Autodesk Fusion 360 part; units mm, degrees
sketch "Esboço1" plane through (0, 0, 0) normal (0, 0, 1) x (1, 0, 0)
  line L0 (0, -15) -> (47.41, -15)
  arc A0 (47.41, -15) -> (47.41, 15) centre (47.41, 0) ccw
  line L1 (47.41, 15) -> (0, 15)
  arc A1 (0, 15) -> (0, -15) centre (0, 0) ccw
  line L2 (0, 0) -> (47.41, 0) construction
  line L3 (-15, 0) -> (62.41, 0) construction
  circle A2 centre (0, 0) radius 3.75
  circle A3 centre (18.25, 0) radius 1.875
  dimension "d1" = 15
  dimension "d4" = 77.41
  dimension "d5" = 7.5
  dimension "d6" = 18.25
  dimension "d7" = 3.75
extrude "Extrusão1" add sketch "Esboço1" along normal blind 5
sketch "Esboço2" plane through (0, 0, 5) normal (0, 0, 1) x (-1, 0, 0)
  circle A0 centre (-18.25, 0) radius 1.875
  circle A1 centre (0, 0) radius 3.75
  arc A2 (0, -15) -> (0, 15) centre (0, 0) ccw
  line L0 (0, 15) -> (-47.41, 15)
  arc A3 (-47.41, 15) -> (-47.41, -15) centre (-47.41, 0) ccw
  line L1 (-47.41, -15) -> (0, -15)
  line L2 (0, 10) -> (-36.5, 10)
  arc A4 (-36.5, 10) -> (-36.5, -10) centre (-36.5, 0) ccw
  line L3 (-36.5, -10) -> (0, -10)
  arc A5 (0, -10) -> (0, 10) centre (0, 0) ccw
  line L4 (0, 0) -> (-36.5, 0) construction
  dimension "d10" = 36.5
  dimension "d11" = 10
extrude "Extrusão2" cut sketch "Esboço2" against normal blind 3.5 contours L2 A4 L3 A5
hole "Furo1" at (36.5, 0, 1.5) direction (0, 0, -1) diameter 10 depth 0.75 tip angle 180
chamfer "Chanfro1" distance 0.75 angle 45 1 edges at (31.8384, 1.8081, 1.5)
chamfer "Chanfro2" distance 5 angle 45 4 edges at (23.705, 15, 0) (-15, 0, 0) (23.705, -15, 0) (62.41, 0, 0)
Build history of the part. All positions in model axes, mm. A direction names the side the tool comes from. Coordinates: 2 decimals unless noted, no trailing zeros. Order: outer loops, then holes, each group sorted by start corner. A loop starts at its lowest first (then second) coordinate and runs counter-clockwise, first axis right, second up. Notation, with made-up numbers: M 12,12 L 27,12 A17 cw 27,37 Z; hole C 5.5,49 d4. An arc over 180 degrees is marked long. One line per question, with ' | ' between items. Start each with the question number.
1. Mould opens along X. For faces 3 (the face through (57.72, -0.23, 0.31)), 4 (the face through (-3.746, -0.165, 0.74)), 5 (the face through (23.2, 10.2, 5)) say: +X half, -X half, draft (parallel to the pull), parting line (faces both ways), or undercut.
2. Wall check: line 1 along X through (y, z) = (-1, 1.2); line 2 along Y through (x, z) = (18.25, 0.65) (3 decimals); line 3 along Z through (x, y) = (9.5, 9.5). Give the ranges that are in metal, low to high. Write a range as [from, to].
3. Tool access for faces 1 (the face through (19, -2, 1.5)), 2 (the face through (23, -13, 3)): list every direction of +Z, -Z, +X, -X, +Y, -Y with a clear straight run to the whole face (end or side of a thin tool).
4. Flat gauge pins, fed straight in: P1, Ø8, axis at x = 36.5, y = 0, coming from the -Z side; P2, Ø1.5, axis at y = 8, z = 1.5, coming from the +X side; P3, Ø3.5, axis at x = 18.25, y = 0, coming from the +Z side; P4, Ø1, axis at x = 8, z = 1.5, coming from the -Y side. Where does each tip first touch, or does it go through?
5. Cut at A-A (y = 0). Count the separate pieces of the cut face and the enclosed holes in it, plus the area to 3 significant figures.
6. Cut at D-D (z = 3.65). Write the cut outline in (x, y), plus the area to 3 significant figures.
The answers:
1) face 3: +X half | face 4: undercut | face 5: draft
2) line 1: x = [-11.16, -3.61], [3.61, 16.66], [19.84, 31.14], [41.86, 58.57] | line 2: y = [-10.651, -1.875], [1.875, 10.651] | line 3: z = [0, 1.5]
3) face 1: +Z | face 2: -Z, +X, -X, -Y
4) P1: stops at z = 0 | P2: stops at x = 56.87 | P3: passes through | P4: stops at y = -12
5) separate pieces: 3 | enclosed holes: 0 | area: 139 mm2
6) outline: M 0,-13.65 L 47.41,-13.65 A13.65 ccw 47.41,13.65 L 0,13.65 A13.65 ccw Z; hole M 0,-10 L 36.5,-10 A10 ccw 36.5,10 L 0,10 A10 ccw Z | area: 836 mm2
